Check sheet for the modelled part. Datum: model origin and axes. Units: mm. A direction names the side the tool comes from. Give positions to 0.01 mm unless a question says otherwise; leave off trailing zeros. Loops run counter-clockwise (first coordinate to the right, second up) from the corner with the lowest first, then second, coordinate; pieces in that order, holes last. Notation, with made-up numbers: (-3, -22.75) - (24, -22.75) arc R21 ccw to (24, -9.75) - close; hole circle Ø10 at (62, -13). An arc over 180 degrees is marked (long way). Use one line per item in the form item = value.
from build123d import *

# Parameters (mm, degrees)
SKETCH_1_W      = 400
SKETCH_1_H      = 300
EXTRUDE_1_DEPTH = 80
SHELL_1_T       = -3
FILLET_1_R      = 3
FILLET_2_R      = 3


with BuildPart() as part:
    # 草图1 → 凸台-拉伸1 (new body)
    with BuildSketch(Plane.XY):
        Rectangle(SKETCH_1_W, SKETCH_1_H)
    extrude(amount=EXTRUDE_1_DEPTH)

    # 抽壳1
    shell_1_openings = [part.faces().sort_by_distance(p)[0] for p in [
        (0, 0, 80),
    ]]
    offset(amount=SHELL_1_T, openings=shell_1_openings, kind=Kind.INTERSECTION)

    # 圆角1
    fillet_1_edges = [part.edges().sort_by_distance(p)[0] for p in [
        (197, 0, 3),
        (197, -147, 41.5),
        (0, 147, 3),
        (197, 147, 41.5),
        (-197, 0, 3),
        (-197, 147, 41.5),
        (0, -147, 3),
        (-197, -147, 41.5),
    ]]
    fillet(fillet_1_edges, radius=FILLET_1_R)

    # 圆角2
    fillet_2_edges = [part.edges().sort_by_distance(p)[0] for p in [
        (200, -150, 40),
        (-200, -150, 40),
        (-200, 150, 40),
        (200, 150, 40),
    ]]
    fillet(fillet_2_edges, radius=FILLET_2_R)


solid = part.part
Item 1: Section check A-A on z = 19.5. Record the boundary of the cut face in (x, y), then the cut area to 3 significant figures.
Answer block:
outline = (-200, -147) arc R3 ccw to (-197, -150) - (197, -150) arc R3 ccw to (200, -147) - (200, 147) arc R3 ccw to (197, 150) - (-197, 150) arc R3 ccw to (-200, 147) - close; hole (-197, -144) arc R3 ccw to (-194, -147) - (194, -147) arc R3 ccw to (197, -144) - (197, 144) arc R3 ccw to (194, 147) - (-194, 147) arc R3 ccw to (-197, 144) - close
area = 4,160 mm2
Item 2: Section check B-B on x = -19. Record the boundary of the cut face in (y, z), then the cut area to 3 significant figures.
Answer block:
outline = (-150, 0) - (150, 0) - (150, 80) - (147, 80) - (147, 6) arc R3 cw to (144, 3) - (-144, 3) arc R3 cw to (-147, 6) - (-147, 80) - (-150, 80) - close
area = 1,370 mm2
Item 3: Section check C-C on y = 35. Record the boundary of the cut face in (x, z), then the cut area to 3 significant figures.
Answer block:
outline = (-200, 0) - (200, 0) - (200, 80) - (197, 80) - (197, 6) arc R3 cw to (194, 3) - (-194, 3) arc R3 cw to (-197, 6) - (-197, 80) - (-200, 80) - close
area = 1,670 mm2
Item 4: Thickness scan on L1, parallel to X at y = -43, z = 10; L2, parallel to Y at x = 43.5, z = 7.5; L3, parallel to Z at x = 22, y = -98. Record the ranges inside material, lowest first.
Answer block:
L1 = -200 to -197, 197 to 200
L2 = -150 to -147, 147 to 150
L3 = 0 to 3
Item 5: Mould release check, pull along X, two halves, no side actions. Record for faces 3 (the face through (200, -2, 39)), 4 (the face through (-197, -2, 42)), 5 (the face through (-3, -150, 39)): released by +X, released by -X, zero draft, split by the parting line, or undercut.
Answer block:
face_3 = released by +X
face_4 = undercut
face_5 = zero draft
Item 6: Access from +Z, -Z, +X, -X, +Y, -Y to the whole of each face (thin tool, end or side, straight path). Record for faces 1 (the face through (197, -2, 42)), 2 (the face through (-3, 2, 0)).
Answer block:
face_1 = +Z
face_2 = -Z, +X, -X, +Y, -Y
